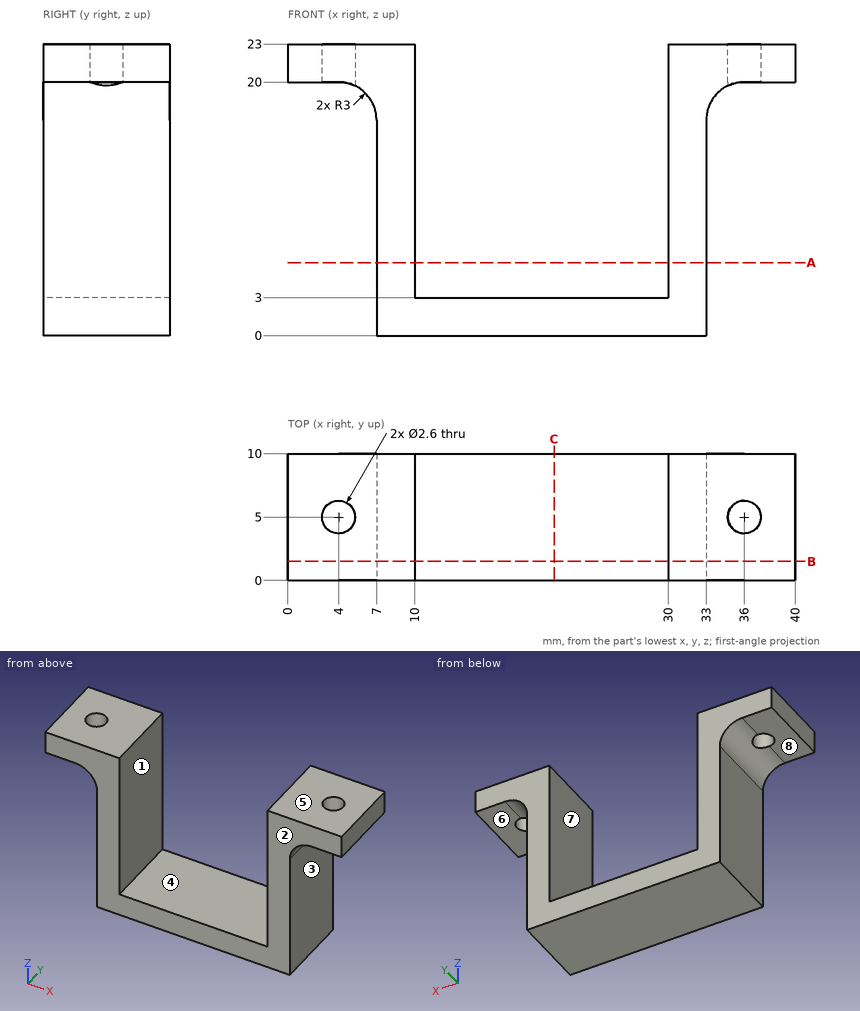
Study the drawing (mm; zero at the part's minimum x, y, z) and answer. A direction names the side the tool comes from. Give positions to 0.01 mm unless a question says otherwise; leave off trailing zeros. Loops run counter-clockwise (first coordinate to the right, second up) from the corner with the lowest first, then second, coordinate; pieces in that order, holes last. Notation, with made-up numbers: M 43,-29.75 L 87,-29.75 A18 cw 87,-17.75 Z; hole C 8,82.25 d5. An arc over 180 degrees is marked long. One line per item, written item: value.
1. Section A-A on z = 5.75 is taken. Determine the outline of the cut face in (x, y), plus the area to 3 significant figures.
Found:
outline: M 7,0 L 10,0 L 10,10 L 7,10 Z; M 30,0 L 33,0 L 33,10 L 30,10 Z
area: 60.0 mm^2
2. For the marked faces 5, 6, 7 and 8, determine the directions among +Z, -Z, +X, -X, +Y, -Y from which every point of the face is accessible in a straight line to the end or side of a thin tool.
Found:
face 5: +Z, +X, -X, +Y, -Y
face 6: -Z, +X, +Y, -Y
face 7: +Z, +Y, -Y
face 8: -Z, -X, +Y, -Y
3. For a pull along X with two mould halves and no side action, classify the marked faces 1, 2, 3 and 4 as pulls with the +X half, pulls with the -X half, needs draft (parallel to the pull), parting line crosses it, or undercut.
Found:
face 1: undercut
face 2: needs draft
face 3: pulls with the +X half
face 4: undercut
4. Find the intervals of material crossed by probe 1 along Y at (x, z) = (4, 21.5); probe 2 along X at (y, z) = (1.5, 21.25); probe 3 along X at (y, z) = (2.5, 15), in increasing order.
Found:
probe 1: 0 to 3.7, 6.3 to 10
probe 2: 0 to 10, 30 to 40
probe 3: 7 to 10, 30 to 33
5. Each of these flat-tipped pins is pushed along its axis until it touches: P1, Ø5, axis at x = 19.5, y = 2.5, coming from the +Z side; P2, Ø3, axis at x = 37.5, y = 5.5, coming from the -Z side; P3, Ø4, axis at x = 36, y = 5, coming from the -Z side. Where does it stop, or does it pass through?
Found:
P1: z = 3
P2: z = 20
P3: z = 19.24
6. Section C-C on x = 21 is taken. Determine the outline of the cut face in (y, z), plus the area to 3 significant figures.
Found:
outline: M 0,0 L 10,0 L 10,3 L 0,3 Z
area: 30.0 mm^2
7. Section B-B on y = 1.5 is taken. Determine the outline of the cut face in (x, z).
Found:
outline: M 0,20 L 4,20 A3 cw 7,17 L 7,0 L 33,0 L 33,17 A3 cw 36,20 L 40,20 L 40,23 L 30,23 L 30,3 L 10,3 L 10,23 L 0,23 Z
